Here's how the part is built. I have some questions about the finished solid (model axes, mm). Face numbers are marked on the shaded views. A direction names the side the tool comes from. Round coordinates to 2 decimals unless told otherwise and drop trailing zeros. Order: outer loops, then holes, each group sorted by start corner. A loop starts at its lowest first (then second) coordinate and runs counter-clockwise, first axis right, second up. Notation, with made-up numbers: (-16, -7.5) -> (2, -7.5) arc R14 cw to (2, 7.5) -> close; hole circle Ø3 at (-24.75, 49.5). An arc over 180 degrees is marked (long way). One line per item, written item: value.
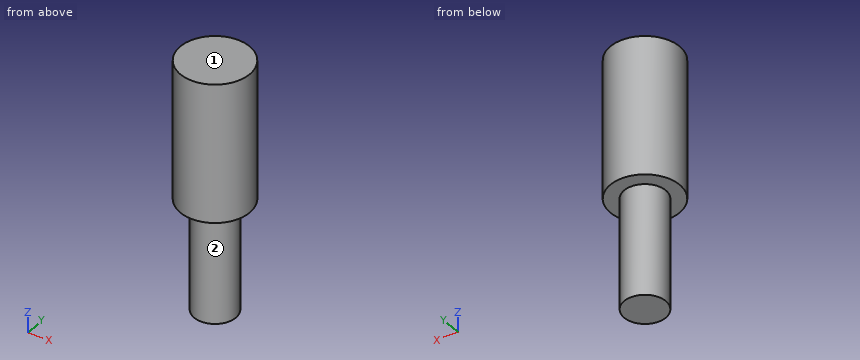
```python
from build123d import *

# Parameters (mm, degrees)
SKETCH_1_R          = 25
EXTRUDE_1_DEPTH     = 100
SKETCH_2_R          = 15
EXTRUDE_2_DEPTH     = 80
SKETCH_3_W          = 8
SKETCH_3_H          = 30
CUT_EXTRUDE_1_DEPTH = 4


with BuildPart() as part:
    # 草图1 → 凸台-拉伸1 (new body)
    with BuildSketch(Plane.XY):
        Circle(SKETCH_1_R)
    extrude(amount=EXTRUDE_1_DEPTH)

    # 草图2 → 凸台-拉伸2 (add)
    with BuildSketch(Plane.XY):
        Circle(SKETCH_2_R)
    extrude(amount=-EXTRUDE_2_DEPTH)

    # 草图3 → 切除-拉伸1 (cut)
    with BuildSketch(Plane(origin=(0, 0, 0), x_dir=(1, 0, 0), z_dir=(0, 1, 0))):
        with Locations((0, -35)):
            Rectangle(SKETCH_3_W, SKETCH_3_H)
    extrude(amount=CUT_EXTRUDE_1_DEPTH, mode=Mode.SUBTRACT)


solid = part.part
```
Q1. Which directions (+Z, -Z, +X, -X, +Y, -Y) give clear straight access to the entire face, cutting with the end or side of a thin tool? Please do the marked faces 1 and 2.
Answers:
face 1: +Z, +X, -X, +Y, -Y
face 2: -Z
Q2. I want a section at C-C on y = -7. Write out the boundary of the cut face in (x, z).
Answers:
outline: (-24, 0) -> (-13.27, 0) -> (-13.27, -80) -> (13.27, -80) -> (13.27, 0) -> (24, 0) -> (24, 100) -> (-24, 100) -> close
Q3. I want a section at B-B on z = 31.5. Write out the boundary of the cut face in (x, y), then the cut area to 3 significant figures.
Answers:
outline: circle Ø50 at (0, 0); hole (-4, 0) -> (4, 0) -> (4, 4) -> (-4, 4) -> close
area: 1,930 mm2
Q4. I need wall thicknesses on line 1 along X through (y, z) = (0.5, 44.5) (3 decimals); line 2 along Z through (x, y) = (9.5, 22.5); line 3 along Y through (x, z) = (0, 22). Which ranges of each line are inside material? Lowest first, please.
Answers:
line 1: -24.995 to -4, 4 to 24.995
line 2: 0 to 100
line 3: -25 to 0, 4 to 25
Q5. I want a section at A-A on x = 0. Write out the boundary of the cut face in (y, z).
Answers:
outline: (-25, 0) -> (-15, 0) -> (-15, -80) -> (15, -80) -> (15, 0) -> (25, 0) -> (25, 100) -> (-25, 100) -> close; hole (0, 20) -> (4, 20) -> (4, 50) -> (0, 50) -> close
Q6. For P1, Ø2, axis at y = 6.5, z = 79, coming from the -X side; P2, Ø5, axis at y = -11, z = -6, coming from the -X side; P3, Ø12, axis at y = 17, z = 22, coming from the -X side; P4, Ø4.5, axis at y = 2, z = 36, coming from the -X side, each with a flat end and sliding along its axis, tell me the tip position at first contact or that it passes through.
Answers:
P1: x = -24.39
P2: x = -12.36
P3: x = -22.45
P4: x = -25
Q7. I want a section at D-D on x = 20. Write out the boundary of the cut face in (y, z).
Answers:
outline: (-15, 0) -> (15, 0) -> (15, 100) -> (-15, 100) -> close
